The listing builds one solid part. Answer for the finished solid, in the listing's coordinates (mm). A direction names the side the tool comes from. Round coordinates to 2 decimals unless told otherwise and drop trailing zeros. Write each loop counter-clockwise with the first axis right and the second up, starting at its lowest first coordinate (ties: lowest second). Pieces come first, ordered by that corner, then holes.
Item 1: Find the intervals of material crossed by probe 1 along Y at (x, z) = (-12, 1); probe 2 along X at (y, z) = (-8, 6.5); probe 3 along X at (y, z) = (-51, 0.25), in increasing order.
Item 2: Each of these flat-tipped pins is pushed along its axis until it touches: pin 1 (2.5 mm diameter, centred on x = -12, y = -50, fed in from +Z); pin 2 (6 mm diameter, centred on x = 12.5, y = -46.5, fed in from -Z). Where does it stop, or does it pass through?
Item 3: Find section C-C on x = 0. Give the vertices of the cut face in (y, z), then the cut area to 3 significant figures.
Item 4: Find section A-A on y = -8. Give the vertices of the cut face in (x, z).
Item 5: Find section B-B on x = 12. Give the vertices of the cut face in (y, z), then the cut area to 3 significant figures.
Item 6: A tool of negligible diameter and unlimited length cuts with its end or side. For faces 1 (the face through (-13, -29, -7)), 2 (the face through (13, -29, -7)), 3 (the face through (0, 0, 5)), from which of +Z, -Z, +X, -X, +Y, -Y can it reach the whole face along a straight path? Write none if from no direction.
Item 7: Find section D-D on y = -15.5. Give the vertices of the cut face in (x, z).
Item 8: For a pull along Y with two mould halves and no side action, classify faces 4 (the face through (-0.867, -28.594, -3.905)), 5 (the face through (-10.43, -8.65, 2.13)), 6 (the face through (0, -58, 5)), 7 (the face through (-11.2, -51.5, 2.1)) as +Y half, -Y half, draft (parallel to the pull), parting line (faces both ways), or undercut.
```python
from build123d import *

# Parameters (mm, degrees)
F0_R     = 4
F1_DEPTH = 58
F2_R     = 1.7
F3_DEPTH = 11.001
F4_DEPTH = 11.001
F5_DEPTH = 50


# Not quite as in the source:
# - a feature names something its author has since deleted; it is built from what else it names


with BuildPart() as f1:
    # F0 (on Front) → F1 (new body)
    with BuildSketch(Plane.XZ):
        with BuildLine():
            Line((-17, -7), (-8.4852813742, -7))
            ThreePointArc((-8.4852813742, -7), (0, -11), (8.4852813742, -7))
            Line((8.4852813742, -7), (17, -7))
            Line((17, -7), (17, 11))
            Line((17, 11), (-17, 11))
            Line((-17, 11), (-17, -7))
        make_face()
        Circle(F0_R, mode=Mode.SUBTRACT)
    extrude(amount=F1_DEPTH)

    # F2 (on Top) → F3 (cut, through all)
    with BuildSketch(Plane.XY):
        with Locations((-12, -8)):
            Circle(F2_R)
        with Locations((12, -8)):
            Circle(F2_R)
        with Locations((12, -50)):
            Circle(F2_R)
        with Locations((-12, -50)):
            Circle(F2_R)
    extrude(amount=-F3_DEPTH, mode=Mode.SUBTRACT)

    # F2 (on Top) → F4 (cut, through all)
    with BuildSketch(Plane.XY):
        with Locations((-12, -8)):
            Circle(F2_R)
        with Locations((12, -8)):
            Circle(F2_R)
        with Locations((12, -50)):
            Circle(F2_R)
        with Locations((-12, -50)):
            Circle(F2_R)
    extrude(amount=-F4_DEPTH, mode=Mode.SUBTRACT)

    # F2 (on Top) → F5 (cut)
    with BuildSketch(Plane.XY):
        with Locations((-12, -8)):
            Circle(F2_R)
        with Locations((12, -8)):
            Circle(F2_R)
        with Locations((12, -50)):
            Circle(F2_R)
        with Locations((-12, -50)):
            Circle(F2_R)
    extrude(amount=F5_DEPTH, mode=Mode.SUBTRACT)


solid = f1.part
```
Check values:
1. probe 1: y = -58 to -51.7, -48.3 to -9.7, -6.3 to 0
1. probe 2: x = -17 to -13.7, -10.3 to 10.3, 13.7 to 17
1. probe 3: x = -17 to -13.37, -10.63 to -3.99, 3.99 to 10.63, 13.37 to 17
2. pin 1: passes through
2. pin 2: stops at z = -7
3. outline: (-58, -11) - (0, -11) - (0, -4) - (-58, -4) - close; (-58, 4) - (0, 4) - (0, 11) - (-58, 11) - close
3. area: 812 mm2
4. outline: (-17, -7) - (-13.7, -7) - (-13.7, 11) - (-17, 11) - close; (-10.3, -7) - (-8.49, -7) arc R11 ccw to (8.49, -7) - (10.3, -7) - (10.3, 11) - (-10.3, 11) - close; (13.7, -7) - (17, -7) - (17, 11) - (13.7, 11) - close; hole circle Ø8 at (0, 0)
5. outline: (-58, -7) - (-51.7, -7) - (-51.7, 11) - (-58, 11) - close; (-48.3, -7) - (-9.7, -7) - (-9.7, 11) - (-48.3, 11) - close; (-6.3, -7) - (0, -7) - (0, 11) - (-6.3, 11) - close
5. area: 922 mm2
6. face 1: -Z, -X, +Y, -Y
6. face 2: -Z, +X, +Y, -Y
6. face 3: +Z, -Z, +X, -X, +Y
7. outline: (-17, -7) - (-8.49, -7) arc R11 ccw to (8.49, -7) - (17, -7) - (17, 11) - (-17, 11) - close; hole circle Ø8 at (0, 0)
8. face 4: draft
8. face 5: undercut
8. face 6: -Y half
8. face 7: undercut
